```python
from build123d import *

# Parameters (mm, degrees)
BASE_EXTRUDE_DEPTH = 101.6
HOLE1_START        = -38.1
HOLE1_OUTLINE_R    = 7.14375
HOLE1_DEPTH        = 2.6924
LPATTERN2_COUNT    = 2
LPATTERN2_PITCH    = 47.625


# Read off the part's stored shape, not the designer's step: Hole1
with BuildPart() as part:
    # Sketch1 → Base-Extrude (new body)
    with BuildSketch(Plane.XY):
        with BuildLine():
            Line((-20.6375, 39.6875), (-20.6375, -35.4076))
            ThreePointArc((-20.6375, -35.4076), (-19.848914298, -37.311414298), (-17.9451, -38.1))
            Line((-17.9451, -38.1), (17.9451, -38.1))
            ThreePointArc((17.9451, -38.1), (19.848914298, -37.311414298), (20.6375, -35.4076))
            Line((20.6375, -35.4076), (20.6375, 39.6875))
            ThreePointArc((20.6375, 39.6875), (15.875, 44.45), (11.1125, 39.6875))
            Line((11.1125, 39.6875), (11.1125, 38.65245))
            ThreePointArc((11.1125, 38.65245), (12.4587, 37.30625), (13.8049, 38.65245))
            Line((13.8049, 38.65245), (13.8049, 39.6875))
            ThreePointArc((13.8049, 39.6875), (15.875, 41.7576), (17.9451, 39.6875))
            Line((17.9451, 39.6875), (17.9451, -35.4076))
            Line((17.9451, -35.4076), (-17.9451, -35.4076))
            Line((-17.9451, -35.4076), (-17.9451, 39.6875))
            ThreePointArc((-17.9451, 39.6875), (-15.875, 41.7576), (-13.8049, 39.6875))
            Line((-13.8049, 39.6875), (-13.8049, 38.65245))
            ThreePointArc((-13.8049, 38.65245), (-12.4587, 37.30625), (-11.1125, 38.65245))
            Line((-11.1125, 38.65245), (-11.1125, 39.6875))
            ThreePointArc((-11.1125, 39.6875), (-15.875, 44.45), (-20.6375, 39.6875))
        make_face()
    extrude(amount=BASE_EXTRUDE_DEPTH)

    # Hole1 outline → Hole1 (cut)
    with BuildSketch(Plane(origin=(0, 0, 0), x_dir=(1, 0, 0), z_dir=(0, 1, 0)).offset(HOLE1_START)):
        with Locations((0, -23.8125)):
            Circle(HOLE1_OUTLINE_R)
    hole1 = extrude(amount=HOLE1_DEPTH, mode=Mode.SUBTRACT)

    # LPattern2: Hole1 ×2
    with Locations(*[(0, 0, i * LPATTERN2_PITCH) for i in range(1, LPATTERN2_COUNT)]):
        add(hole1, mode=Mode.SUBTRACT)


solid = part.part
```
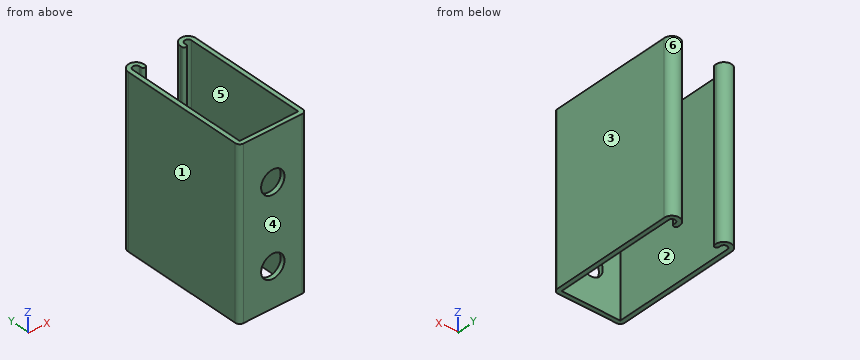
Model file for the job. Use its own axes, mm. Face numbers are marked on the shaded views. A direction names the side the tool comes from. Round coordinates to 2 decimals unless told otherwise and drop trailing zeros. Loops run counter-clockwise (first coordinate to the right, second up) from the corner with the lowest first, then second, coordinate; pieces in that order, holes last. Notation, with made-up numbers: M -6,32 L 21,32 A21 ccw 21,53 Z; hole C -24.5,20 d4. An arc over 180 degrees is marked long. Put each result on its own line as item: value. Start each with the question number.
Item 1: 3-axis set-ups, long thin cutter, end or side, ignore diameter. For the marked faces 1 and 2: which of +Z, -Z, +X, -X, +Y, -Y reach the whole face in a straight line?
Item 2: Cut at C-C (z = 94). List the corners of the cut face in (x, y) (1 decimal), then the cut area to 3 significant figures.
Item 3: Drop a flat-ended pin along its axis: P1, Ø16.5, axis at x = 0, z = 71.44, coming from the +Y side. Give the stop position or say it passes through.
Item 4: Cut at A-A (x = 0). List the corners of the cut face in (y, z).
Item 5: Cut at D-D (x = -16). List the corners of the cut face in (y, z).
Item 6: Cut at B-B (y = -13). List the corners of the cut face in (x, z).
Item 7: Drill centre lines: line 1 along Z through (x, y) = (0, -36); line 2 along X through (y, z) = (-12.5, 39); line 3 along Y through (x, z) = (16, 31). Where is each one in solid material? Low to high.
Item 8: Mould opens along Y. For the marked faces 3, 4, 5 and 6 say: released by +Y, released by -Y, zero draft, split by the parting line, or undercut.
Answer block:
1. face 1: +Z, -Z, -X, +Y, -Y
1. face 2: +Z, -Z
2. outline: M -20.6,-35.4 A2.7 ccw -17.9,-38.1 L 17.9,-38.1 A2.7 ccw 20.6,-35.4 L 20.6,39.7 A4.8 ccw 11.1,39.7 L 11.1,38.7 A1.3 ccw 13.8,38.7 L 13.8,39.7 A2.1 cw 17.9,39.7 L 17.9,-35.4 L -17.9,-35.4 L -17.9,39.7 A2.1 cw -13.8,39.7 L -13.8,38.7 A1.3 ccw -11.1,38.7 L -11.1,39.7 A4.8 ccw -20.6,39.7 Z
2. area: 581 mm2
3. P1: y = -35.41
4. outline: M -38.1,0 L -35.41,0 L -35.41,16.67 L -38.1,16.67 Z; M -38.1,30.96 L -35.41,30.96 L -35.41,64.29 L -38.1,64.29 Z; M -38.1,78.58 L -35.41,78.58 L -35.41,101.6 L -38.1,101.6 Z
5. outline: M -38.1,0 L -35.41,0 L -35.41,101.6 L -38.1,101.6 Z; M 41.75,0 L 44.45,0 L 44.45,101.6 L 41.75,101.6 Z
6. outline: M -20.64,0 L -17.95,0 L -17.95,101.6 L -20.64,101.6 Z; M 17.95,0 L 20.64,0 L 20.64,101.6 L 17.95,101.6 Z
7. line 1: 0 to 16.67, 30.96 to 64.29, 78.58 to 101.6
7. line 2: -20.64 to -17.95, 17.95 to 20.64
7. line 3: -38.1 to -35.41, 41.75 to 44.45
8. face 3: zero draft
8. face 4: released by -Y
8. face 5: undercut
8. face 6: released by +Y
